Check sheet for the modelled part. Datum: model origin and axes. Units: mm. Face numbers are marked on the shaded views. Round coordinates to 2 decimals unless told otherwise and drop trailing zeros. Order: outer loops, then holes, each group sorted by start corner. A loop starts at its lowest first (then second) coordinate and runs counter-clockwise, first axis right, second up. Notation, with made-up numbers: (-27.75, 21.5) -> (15.25, 21.5) arc R19 ccw to (15.25, 31.5) -> close; hole circle Ø1 at (57, -17). An arc over 180 degrees is marked (long way). Use CSV: the item, a comma, the result in double quotes.
Autodesk Inventor part; units mm, degrees
ref_plane "YZ Plane" through (0, 0, 0) normal (1, 0, 0) x (0, 1, 0)
ref_plane "XZ Plane" through (0, 0, 0) normal (0, 1, 0) x (-1, 0, 0)
ref_plane "XY Plane" through (0, 0, 0) normal (0, 0, 1) x (1, 0, 0)
sketch "Sketch1" plane through (0, 0, 0) normal (0, 1, 0) x (-1, 0, 0)
  circle A0 centre (0, 0) radius 34
  dimension "d0" = 68
extrude "Extrusion1" add sketch "Sketch1" along normal blind 27
sketch "Sketch2" plane through (0, 27, 0) normal (0, 1, 0) x (1, 0, 0)
  circle A0 centre (0, 0) radius 30
  dimension "d3" = 60
extrude "Extrusion2" cut sketch "Sketch2" against normal blind 12
sketch "Sketch5" plane through (0, 15, 0) normal (0, 1, 0) x (1, 0, 0)
  circle A0 centre (0, 0) radius 2
  dimension "d13" = 4
extrude "Extrusion5" cut sketch "Sketch5" against normal through all
properties part number "Wheel"
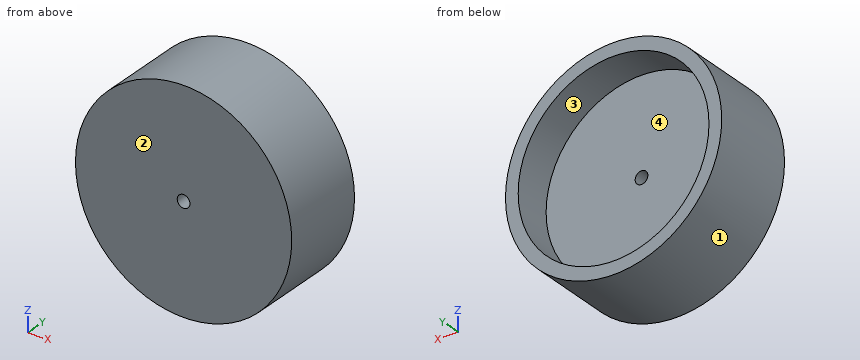
Q1. Sectioned sample at D-D, the plane x = -20.5. Enter the section's corners in (y, z).
Result sheet:
outline,"(0, -27.12) -> (27, -27.12) -> (27, -21.9) -> (15, -21.9) -> (15, 21.9) -> (27, 21.9) -> (27, 27.12) -> (0, 27.12) -> close"
Q2. Sectioned sample at A-A, the plane x = 0. Enter the section's corners in (y, z), then the cut area to 3 significant figures.
Result sheet:
outline,"(0, -34) -> (27, -34) -> (27, -30) -> (15, -30) -> (15, -2) -> (0, -2) -> close; (0, 2) -> (15, 2) -> (15, 30) -> (27, 30) -> (27, 34) -> (0, 34) -> close"
area,"1,060 mm^2"
Q3. Scan lines: L1, parallel to Z at x = 0, y = 24.75; L2, parallel to Z at x = 0, y = 8; L3, parallel to Y at x = 11.5, z = -11. Record each from-to range of solid material in increasing order.
Result sheet:
L1,"z = -34 to -30, 30 to 34"
L2,"z = -34 to -2, 2 to 34"
L3,"y = 0 to 15"
Q4. Sectioned sample at C-C, the plane y = 11.75. Enter the section's corners in (x, z), then the cut area to 3 significant figures.
Result sheet:
outline,"circle Ø68 at (0, 0); hole circle Ø4 at (0, 0)"
area,"3,620 mm^2"
Q5. Mould release check, pull along Z, two halves, no side actions. Record for the marked faces 1, 2, 3 and 4: pulls with the +Z half, pulls with the -Z half, needs draft (parallel to the pull), parting line crosses it, or undercut.
Result sheet:
face 1,"parting line crosses it"
face 2,"needs draft"
face 3,"undercut"
face 4,"undercut"
Q6. Sectioned sample at B-B, the plane z = 0. Enter the section's corners in (x, y), then the cut area to 3 significant figures.
Result sheet:
outline,"(-34, 0) -> (-2, 0) -> (-2, 15) -> (-30, 15) -> (-30, 27) -> (-34, 27) -> close; (2, 0) -> (34, 0) -> (34, 27) -> (30, 27) -> (30, 15) -> (2, 15) -> close"
area,"1,060 mm^2"
Q7. Go/stop test with flat-tipped pins: pin 1 (8 mm diameter, centred on y = 13, z = 7, fed in from -X); pin 2 (1 mm diameter, centred on y = 8.5, z = 22.5, fed in from -X); pin 3 (5 mm diameter, centred on x = 0, z = 0, fed in from +Y). Record where each tip stops, or that it passes through.
Result sheet:
pin 1,"stops at x = -33.87"
pin 2,"stops at x = -25.92"
pin 3,"stops at y = 15"
